from build123d import *

# Parameters (mm, degrees)
SKETCH1_W           = 100
SKETCH1_H           = 100
SKETCH1_R           = 2.5
SKETCH1_R_2         = 29.5
BOSS_EXTRUDE1_DEPTH = 5
SKETCH1_3_R         = 29.5
BOSS_EXTRUDE2_DEPTH = 1
CHAMFER1_SIZE       = 10
CHAMFER3_SIZE       = 1.5


with BuildPart() as part:
    # Sketch1 → Boss-Extrude1 (new body)
    with BuildSketch(Plane(origin=(0, 0, 0), x_dir=(1, 0, 0), z_dir=(0, 1, 0))):
        Rectangle(SKETCH1_W, SKETCH1_H)
        with Locations((40, -40)):
            Circle(SKETCH1_R, mode=Mode.SUBTRACT)
        with Locations((-40, 40)):
            Circle(SKETCH1_R, mode=Mode.SUBTRACT)
        Circle(SKETCH1_R_2, mode=Mode.SUBTRACT)
        with Locations((40, 40)):
            Circle(SKETCH1_R, mode=Mode.SUBTRACT)
        with Locations((-40, -40)):
            Circle(SKETCH1_R, mode=Mode.SUBTRACT)
    extrude(amount=BOSS_EXTRUDE1_DEPTH)

    # Sketch1<3> → Boss-Extrude2 (add)
    with BuildSketch(Plane(origin=(0, 0, 0), x_dir=(1, 0, 0), z_dir=(0, 1, 0))):
        Circle(SKETCH1_3_R)
    extrude(amount=BOSS_EXTRUDE2_DEPTH)

    # Chamfer1
    chamfer1_edges = [part.edges().sort_by_distance(p)[0] for p in [
        (-50, 2.5, 50),
        (-50, 2.5, -50),
        (50, 2.5, -50),
        (50, 2.5, 50),
    ]]
    chamfer(chamfer1_edges, length=CHAMFER1_SIZE)

    # Chamfer3
    chamfer3_edges = [part.edges().sort_by_distance(p)[0] for p in [
        (37.5, 5, 40),
        (-42.5, 5, -40),
        (37.5, 5, -40),
        (-42.5, 5, 40),
    ]]
    chamfer(chamfer3_edges, length=CHAMFER3_SIZE)


solid = part.part
Geometry check sheet. Reference: the model listing, model coordinates, mm. Round coordinates to 2 decimals unless told otherwise and drop trailing zeros. Write each loop counter-clockwise with the first axis right and the second up, starting at its lowest first coordinate (ties: lowest second). Pieces come first, ordered by that corner, then holes. Notation, with made-up numbers: (28, 87) - (54, 87) arc R29 cw to (54, 124) - close; hole circle Ø10 at (-24.5, -6). An arc over 180 degrees is marked (long way). One line per item, written item: value.
1. Cross-section at C-C on x = -4. Record the boundary of the cut face in (y, z).
The answers:
outline: (0, -50) - (5, -50) - (5, -29.23) - (1, -29.23) - (1, 29.23) - (5, 29.23) - (5, 50) - (0, 50) - close
2. Cross-section at B-B on z = 0. Record the boundary of the cut face in (x, y).
The answers:
outline: (-50, 0) - (50, 0) - (50, 5) - (29.5, 5) - (29.5, 1) - (-29.5, 1) - (-29.5, 5) - (-50, 5) - close
3. Mould release check, pull along Z, two halves, no side actions. Record for faces 1 (the face through (45, 2, 45)), 2 (the face through (-37.69, 1.73, -39.04)), 3 (the face through (-45, 2, -45)): released by +Z, released by -Z, zero draft, split by the parting line, or undercut.
The answers:
face 1: released by +Z
face 2: undercut
face 3: released by -Z
4. Scan lines: L1, parallel to Z at x = -40, y = 0.9; L2, parallel to Z at x = 41.5, y = 1.9. Record each from-to range of solid material in increasing order.
The answers:
L1: z = -50 to -42.5, -37.5 to 37.5, 42.5 to 50
L2: z = -48.5 to -42, -38 to 38, 42 to 48.5
5. Cross-section at A-A on y = 2.3. Record the boundary of the cut face in (x, z).
The answers:
outline: (-50, -40) - (-40, -50) - (40, -50) - (50, -40) - (50, 40) - (40, 50) - (-40, 50) - (-50, 40) - close; hole circle Ø5 at (-40, -40); hole circle Ø5 at (-40, 40); hole circle Ø59 at (0, 0); hole circle Ø5 at (40, -40); hole circle Ø5 at (40, 40)
